```python
from build123d import *

# Parameters (mm, degrees)
SKETCH1_R           = 120
BOSS_EXTRUDE1_DEPTH = 40
BOSS_EXTRUDE2_START = 40
SKETCH1_3_R         = 110
BOSS_EXTRUDE2_DEPTH = 20
CUT_EXTRUDE1_START  = 60
SKETCH1_5_R         = 105
SKETCH1_5_R_2       = 100
CUT_EXTRUDE1_DEPTH  = 10
SKETCH2_R           = 16
CUT_EXTRUDE2_DEPTH  = 10


with BuildPart() as part:
    # Sketch1 → Boss-Extrude1 (new body)
    with BuildSketch(Plane(origin=(0, 0, 0), x_dir=(1, 0, 0), z_dir=(0, 1, 0))):
        with Locations(Location((0, 0, 0), (0, 0, 270))):
            Circle(SKETCH1_R)
    extrude(amount=BOSS_EXTRUDE1_DEPTH)

    # Sketch1<3> → Boss-Extrude2 (add)
    with BuildSketch(Plane(origin=(0, 0, 0), x_dir=(1, 0, 0), z_dir=(0, 1, 0)).offset(BOSS_EXTRUDE2_START)):
        with Locations(Location((0, 0, 0), (0, 0, 270))):
            Circle(SKETCH1_3_R)
    extrude(amount=BOSS_EXTRUDE2_DEPTH)

    # Sketch1<5> → Cut-Extrude1 (cut)
    with BuildSketch(Plane(origin=(0, 0, 0), x_dir=(1, 0, 0), z_dir=(0, 1, 0)).offset(CUT_EXTRUDE1_START)):
        with Locations(Location((0, 0, 0), (0, 0, 270))):
            Circle(SKETCH1_5_R)
        with Locations(Location((0, 0, 0), (0, 0, 270))):
            Circle(SKETCH1_5_R_2, mode=Mode.SUBTRACT)
    extrude(amount=-CUT_EXTRUDE1_DEPTH, mode=Mode.SUBTRACT)

    # Sketch2 → Cut-Extrude2 (cut)
    with BuildSketch(Plane(origin=(0, 60, 0), x_dir=(1, 0, 0), z_dir=(0, 1, 0))):
        with Locations(Location((0, 0, 0), (0, 0, 270))):
            Circle(SKETCH2_R)
    extrude(amount=-CUT_EXTRUDE2_DEPTH, mode=Mode.SUBTRACT)


solid = part.part
```
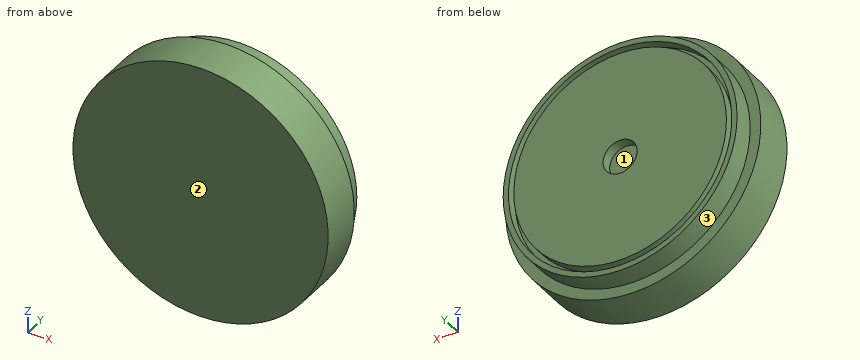
For this review, take the finished solid that the model builds, in its own axes (mm). Face numbers are marked on the shaded views. Coordinates: 2 decimals unless noted, no trailing zeros. Write each loop counter-clockwise with the first axis right and the second up, starting at its lowest first coordinate (ties: lowest second). Pieces come first, ordered by that corner, then holes.
(1) For pin 1 Ø1.5 at (x, y) = (2, 18) entering from +Z; pin 2 Ø8 at (x, y) = (37.5, 25) entering from -Z; pin 3 Ø8 at (x, y) = (-51.5, 38.5) entering from +Z, all flat-tipped, find the tip position at first contact; note any pin that passes through.
(2) Add section B-B on z = 0. Give the boundary of the cut face in (x, y), then the cut area to 3 significant figures.
(3) Add section C-C on y = 25.5. Give the boundary of the cut face in (x, z), then the cut area to 3 significant figures.
(4) Wall thickness on probe 1 along X at (y, z) = (54, 0); probe 2 along Z at (x, y) = (-74.5, 54); probe 3 along X at (y, z) = (54, -64.5): over which ranges is each line inside the solid? List them lowest first.
(5) The part is to be moulded in two halves that separate along Z. For the marked faces 1, 2 and 3, say which applies: +Z half, -Z half, draft (parallel to the pull), parting line (faces both ways), or undercut.
(6) Add section A-A on x = 0. Give the boundary of the cut face in (y, z).
(7) Add section D-D on x = -94.5. Give the boundary of the cut face in (y, z).
Answer sheet:
1. pin 1: stops at z = 119.99
1. pin 2: stops at z = -115.23
1. pin 3: stops at z = 110.2
2. outline: (-120, 0) - (120, 0) - (120, 40) - (110, 40) - (110, 60) - (105, 60) - (105, 50) - (100, 50) - (100, 60) - (16, 60) - (16, 50) - (-16, 50) - (-16, 60) - (-100, 60) - (-100, 50) - (-105, 50) - (-105, 60) - (-110, 60) - (-110, 40) - (-120, 40) - close
2. area: 13,600 mm2
3. outline: circle Ø240 at (0, 0)
3. area: 45,200 mm2
4. probe 1: x = -110 to -105, -100 to -16, 16 to 100, 105 to 110
4. probe 2: z = -80.93 to -73.99, -66.71 to 66.71, 73.99 to 80.93
4. probe 3: x = -89.11 to -82.85, -76.42 to 76.42, 82.85 to 89.11
5. face 1: undercut
5. face 2: draft
5. face 3: parting line
6. outline: (0, -120) - (40, -120) - (40, -110) - (60, -110) - (60, -105) - (50, -105) - (50, -100) - (60, -100) - (60, -16) - (50, -16) - (50, 16) - (60, 16) - (60, 100) - (50, 100) - (50, 105) - (60, 105) - (60, 110) - (40, 110) - (40, 120) - (0, 120) - close
7. outline: (0, -73.96) - (40, -73.96) - (40, -56.3) - (60, -56.3) - (60, -45.77) - (50, -45.77) - (50, -32.71) - (60, -32.71) - (60, 32.71) - (50, 32.71) - (50, 45.77) - (60, 45.77) - (60, 56.3) - (40, 56.3) - (40, 73.96) - (0, 73.96) - close
